Input: part model. Units: mm. Frame: model coordinates. A direction names the side the tool comes from. Coordinates: 2 decimals unless noted, no trailing zeros. Order: outer loops, then holes, each group sorted by start corner. A loop starts at its lowest first (then second) coordinate and runs counter-clockwise, first axis right, second up. Notation, with made-up numbers: M 89,32 L 121,32 A14 ccw 121,51 Z; hole C 69,-33.75 d3. An arc over 180 degrees is marked long. Answer in a Markdown table with one row per item.
from build123d import *

# Parameters (mm, degrees)
F1_DEPTH = 150
F2_W     = 12
F2_H     = 6
F3_DEPTH = 108.3


with BuildPart() as f1:
    # F0 (on Right) → F1 (new body)
    with BuildSketch(Plane.YZ):
        Polygon((0, 55), (0, 0), (12, 0), (12, 68), (0, 68), (0, 58), (3, 58), (3, 55), align=None)
    extrude(amount=F1_DEPTH)

    # F2 (on face) → F3 (cut)
    with BuildSketch(Plane.XY.offset(68)):
        with Locations((6, 3)):
            Rectangle(F2_W, F2_H)
        with Locations((144, 3)):
            Rectangle(F2_W, F2_H)
    extrude(amount=-F3_DEPTH, mode=Mode.SUBTRACT)


solid = f1.part
1) Contact query for flat-ended pins moving along their axis: pin 1 (2 mm diameter, centred on y = 2, z = 16, fed in from -X); pin 2 (1.5 mm diameter, centred on x = 80.5, z = 56, fed in from -Y); pin 3 (5 mm diameter, centred on y = 2, z = 45.5, fed in from +X). Output: stop coordinate, or through.
Resolved:
| item | result |
|---|---|
| pin 1 | stops at x = 12 |
| pin 2 | stops at y = 3 |
| pin 3 | stops at x = 138 |
2) Cut plane A-A, the plane y = 1.5. Output: boundary loops of the cut face in (x, z).
Resolved:
| item | result |
|---|---|
| outline | M 12,0 L 138,0 L 138,55 L 12,55 Z; M 12,58 L 138,58 L 138,68 L 12,68 Z |
3) Reachability of faces 1 (the face through (74, 6, 68)), 2 (the face through (12, 3, 34)), 3 (the face through (74, 3, 57)), 4 (the face through (138, 3, 34)) from +Z, -Z, +X, -X, +Y, -Y: full face, straight path, thin tool, end or side. Return the list, or none.
Resolved:
| item | result |
|---|---|
| face 1 | +Z, +X, -X, +Y, -Y |
| face 2 | +Z, -Z, -X, -Y |
| face 3 | +X, -X, -Y |
| face 4 | +Z, -Z, +X, -Y |
4) Material intervals for probe 1 along Z at (x, y) = (119.5, 1); probe 2 along X at (y, z) = (5.5, 3); probe 3 along Y at (x, z) = (7.5, 22), sorted ascending.
Resolved:
| item | result |
|---|---|
| probe 1 | z = 0 to 55, 58 to 68 |
| probe 2 | x = 12 to 138 |
| probe 3 | y = 6 to 12 |
5) Mould query, pull axis Z, two halves, no side actions, for faces 5 (the face through (74, 2, 55)), 6 (the face through (74, 1, 58)), 7 (the face through (144, 6, 34)), 8 (the face through (74, 6, 0)). Classes: +Z half, -Z half, draft (parallel to the pull), parting line (faces both ways), or undercut.
Resolved:
| item | result |
|---|---|
| face 5 | undercut |
| face 6 | undercut |
| face 7 | draft |
| face 8 | -Z half |
6) Cut plane B-B, the plane z = 5. Output: boundary loops of the cut face in (x, y), and give its area (3 significant figures).
Resolved:
| item | result |
|---|---|
| outline | M 0,6 L 12,6 L 12,0 L 138,0 L 138,6 L 150,6 L 150,12 L 0,12 Z |
| area | 1,660 mm2 |
